Here's how the part is built. I have some questions about the finished solid (model axes, mm). A direction names the side the tool comes from. Round coordinates to 2 decimals unless told otherwise and drop trailing zeros. Loops run counter-clockwise (first coordinate to the right, second up) from the corner with the lowest first, then second, coordinate; pieces in that order, holes last. Notation, with made-up numbers: M -30,15 L -17,15 A31 cw -17,40 Z; hole C 1.5,26.5 d2. An arc over 180 degrees is marked long. Answer as CSV lines item,"result".
```python
from build123d import *
from build123d.topology import SkipClean

# Parameters (mm, degrees)
SKETCH_1_R               = 82.5
SKETCH_1_R_2             = 12.5
EXTRUDE_1_DEPTH          = 5
SKETCH_2_R               = 4
SKETCH_2_R_2             = 3
EXTRUDE_2_DEPTH          = 18
EXTRUDE_START            = 5
SKETCH_3_R               = 35
SKETCH_3_R_2             = 12.5
EXTRUDE_3_DEPTH          = 5
CUT_EXTRUDE_1_DEPTH      = 119.05295422
CUT_EXTRUDE_1_DEPTH_BACK = 10
SKETCH_4_R               = 82.5
EXTRUDE_4_DEPTH          = 5
SKETCH_6_R               = 12.5
CUT_EXTRUDE_2_DEPTH      = 110.399094856
SKETCH_7_R               = 34.75
SKETCH_7_R_2             = 12.5
EXTRUDE_5_DEPTH          = 5


with BuildPart() as part:
    # 草圖1 → 填料-伸長1 (new body)
    with BuildSketch(Plane(origin=(0, 0, 0), x_dir=(1, 0, 0), z_dir=(0, 1, 0))):
        with Locations(Location((0, 0, 0), (0, 0, 270))):
            Circle(SKETCH_1_R)
        with Locations(Location((0, 0, 0), (0, 0, 270))):
            Circle(SKETCH_1_R_2, mode=Mode.SUBTRACT)
    extrude(amount=EXTRUDE_1_DEPTH)

    # 草圖2 → 填料-伸長2 (add)
    # profile 1 of 3: a face of its own
    with BuildSketch(Plane(origin=(0, 5, 0), x_dir=(1, 0, 0), z_dir=(0, 1, 0))):
        with Locations(Location((0, 71.25, 0), (0, 0, 270))):
            Circle(SKETCH_2_R)
        with Locations(Location((0, 71.25, 0), (0, 0, 270))):
            Circle(SKETCH_2_R_2, mode=Mode.SUBTRACT)
    # profile 2 of 3: a face of its own
    with BuildSketch(Plane(origin=(0, 5, 0), x_dir=(1, 0, 0), z_dir=(0, 1, 0))):
        with Locations(Location((61.70431002, -35.625, 0), (0, 0, 270))):
            Circle(SKETCH_2_R)
        with Locations(Location((61.70431002, -35.625, 0), (0, 0, 270))):
            Circle(SKETCH_2_R_2, mode=Mode.SUBTRACT)
    # profile 3 of 3: a face of its own
    with BuildSketch(Plane(origin=(0, 5, 0), x_dir=(1, 0, 0), z_dir=(0, 1, 0))):
        with Locations(Location((-61.70431002, -35.625, 0), (0, 0, 270))):
            Circle(SKETCH_2_R)
        with Locations(Location((-61.70431002, -35.625, 0), (0, 0, 270))):
            Circle(SKETCH_2_R_2, mode=Mode.SUBTRACT)
    extrude(amount=EXTRUDE_2_DEPTH)

    # 草圖3 → 填料-伸長3 (add)
    with SkipClean():  # the faces are left unmerged after this step: merging them gives an invalid solid
        with BuildSketch(Plane.XZ.offset(EXTRUDE_START)):
            with Locations(Location((0, 0, 0), (0, 0, 90))):
                Circle(SKETCH_3_R)
            with Locations(Location((0, 0, 0), (0, 0, 270))):
                Circle(SKETCH_3_R_2, mode=Mode.SUBTRACT)
        extrude(amount=-EXTRUDE_3_DEPTH)

    # 草圖4 → 除料-伸長1 (cut, two sides: drawn at the far end of the back side and taken through both)
    with SkipClean():  # the faces are left unmerged after this step: merging them gives an invalid solid
        with BuildSketch(Plane(origin=(0, 5, 0), x_dir=(1, 0, 0), z_dir=(0, 1, 0)).offset(-CUT_EXTRUDE_1_DEPTH_BACK)):
            Circle(SKETCH_4_R)
            with BuildLine():
                ThreePointArc((-35.334504499, -38.829406277), (0, -52.5), (35.334504499, -38.829406277))
                ThreePointArc((35.334504499, -38.829406277), (40.993396246, -36.283053927), (47.064886308, -37.565229625))
                Line((47.064886308, -37.565229625), (57.20431002, -43.419228634))
                ThreePointArc((57.20431002, -43.419228634), (69.498538654, -40.125), (66.20431002, -27.830771366))
                Line((66.20431002, -27.830771366), (56.064886308, -21.976772357))
                ThreePointArc((56.064886308, -21.976772357), (51.918744551, -17.359795573), (51.294504499, -11.185875388))
                ThreePointArc((51.294504499, -11.185875388), (45.466333699, 26.25), (15.96, 50.015281665))
                ThreePointArc((15.96, 50.015281665), (10.925348305, 53.6428495), (9, 59.542001982))
                Line((9, 59.542001982), (9, 71.25))
                ThreePointArc((9, 71.25), (0, 80.25), (-9, 71.25))
                Line((-9, 71.25), (-9, 59.542001982))
                ThreePointArc((-9, 59.542001982), (-10.925348305, 53.6428495), (-15.96, 50.015281665))
                ThreePointArc((-15.96, 50.015281665), (-45.466333699, 26.25), (-51.294504499, -11.185875388))
                ThreePointArc((-51.294504499, -11.185875388), (-51.918744551, -17.359795573), (-56.064886308, -21.976772357))
                Line((-56.064886308, -21.976772357), (-66.20431002, -27.830771366))
                ThreePointArc((-66.20431002, -27.830771366), (-69.498538654, -40.125), (-57.20431002, -43.419228634))
                Line((-57.20431002, -43.419228634), (-47.064886308, -37.565229625))
                ThreePointArc((-47.064886308, -37.565229625), (-40.993396246, -36.283053927), (-35.334504499, -38.829406277))
            make_face(mode=Mode.SUBTRACT)
        extrude(amount=CUT_EXTRUDE_1_DEPTH + CUT_EXTRUDE_1_DEPTH_BACK, mode=Mode.SUBTRACT)

    # 草圖5 → 填料-伸長4 (add)
    with BuildSketch(Plane.XZ):
        with BuildLine():
            Line((-47.064886308, 37.565229625), (-57.20431002, 43.419228634))
            ThreePointArc((-57.20431002, 43.419228634), (-69.498538654, 40.125), (-66.20431002, 27.830771366))
            Line((-66.20431002, 27.830771366), (-56.064886308, 21.976772357))
            ThreePointArc((-56.064886308, 21.976772357), (-51.918744551, 17.359795573), (-51.294504499, 11.185875388))
            ThreePointArc((-51.294504499, 11.185875388), (-45.466333699, -26.25), (-15.96, -50.015281665))
            ThreePointArc((-15.96, -50.015281665), (-10.925348305, -53.6428495), (-9, -59.542001982))
            Line((-9, -59.542001982), (-9, -71.25))
            ThreePointArc((-9, -71.25), (0, -80.25), (9, -71.25))
            Line((9, -71.25), (9, -59.542001982))
            ThreePointArc((9, -59.542001982), (10.925348305, -53.6428495), (15.96, -50.015281665))
            ThreePointArc((15.96, -50.015281665), (45.466333699, -26.25), (51.294504499, 11.185875388))
            ThreePointArc((51.294504499, 11.185875388), (51.918744551, 17.359795573), (56.064886308, 21.976772357))
            Line((56.064886308, 21.976772357), (66.20431002, 27.830771366))
            ThreePointArc((66.20431002, 27.830771366), (69.498538654, 40.125), (57.20431002, 43.419228634))
            Line((57.20431002, 43.419228634), (47.064886308, 37.565229625))
            ThreePointArc((47.064886308, 37.565229625), (40.993396246, 36.283053927), (35.334504499, 38.829406277))
            ThreePointArc((35.334504499, 38.829406277), (0, 52.5), (-35.334504499, 38.829406277))
            ThreePointArc((-35.334504499, 38.829406277), (-40.993396246, 36.283053927), (-47.064886308, 37.565229625))
        make_face()
    extrude(amount=EXTRUDE_4_DEPTH)

    # 草圖6 → 除料-伸長2 (cut, through all)
    with BuildSketch(Plane(origin=(0, 0, 0), x_dir=(1, 0, 0), z_dir=(0, 1, 0))):
        with Locations(Location((0, 0, 0), (0, 0, 270))):
            Circle(SKETCH_6_R)
    extrude(amount=-CUT_EXTRUDE_2_DEPTH, mode=Mode.SUBTRACT)

    # 草圖7 → 填料-伸長5 (add)
    with SkipClean():  # the faces are left unmerged after this step: merging them gives an invalid solid
        with BuildSketch(Plane.XZ.offset(5)):
            with Locations(Location((0, 0, 0), (0, 0, 270))):
                Circle(SKETCH_7_R)
            with Locations(Location((0, 0, 0), (0, 0, 270))):
                Circle(SKETCH_7_R_2, mode=Mode.SUBTRACT)
        extrude(amount=EXTRUDE_5_DEPTH)
    add(part.part.scale(1), mode=Mode.REPLACE)  # the faces are merged on a copy


solid = part.part
```
1. For P1, Ø8, axis at x = -16.5, z = 15.5, coming from the +Y side; P2, Ø8, axis at x = 0, z = -71.25, coming from the -Y side; P3, Ø11, axis at y = -2, z = -62.5, coming from the +X side; P4, Ø15, axis at x = 0, z = 0, coming from the +Y side, each with a flat end and sliding along its axis, tell me the tip position at first contact or that it passes through.
Evaluation:
P1,"stops at y = 5"
P2,"stops at y = -5"
P3,"stops at x = 9.33"
P4,"passes through"
2. We'd pull the mould along X, two halves only. Please class faces 1 (the cylindrical face through (63.73, 13.87, 33.41)), 2 (the flat face through (9, 0, -65)), 3 (the flat face through (0, -10, -15)), 4 (the cylindrical face through (34.454, -7.465, 4.524)): pulls with the +X half, pulls with the -X half, needs draft (parallel to the pull), parting line crosses it, or undercut.
Evaluation:
face 1,"undercut"
face 2,"pulls with the +X half"
face 3,"needs draft"
face 4,"parting line crosses it"
3. If I drill on line 1 (X direction, y = -6.65, z = 0); line 2 (X direction, y = 1, z = 42.5); line 3 (Z direction, x = 0, y = -3.8), over which ranges is the centre line in solid material (lowest first)? Write a range as [from, to].
Evaluation:
line 1,"x = [-34.75, -12.5], [12.5, 34.75]"
line 2,"x = [-67.51, -55.61], [-30.82, 30.82], [55.61, 67.51]"
line 3,"z = [-80.25, -12.5], [12.5, 52.5]"
4. I want a section at B-B, the plane z = 0. Please give me the cut outline in (x, y).
Evaluation:
outline,"M -52.5,-5 L -34.75,-5 L -34.75,-10 L -12.5,-10 L -12.5,5 L -52.5,5 Z; M 12.5,-10 L 34.75,-10 L 34.75,-5 L 52.5,-5 L 52.5,5 L 12.5,5 Z"
5. I want a section at D-D, the plane x = -24. Please give me the cut outline in (y, z), and give its area (3 significant figures).
Evaluation:
outline,"M -10,-25.13 L -5,-25.13 L -5,-46.69 L 5,-46.69 L 5,46.69 L -5,46.69 L -5,25.13 L -10,25.13 Z"
area,"1,190 mm²"
6. I want a section at A-A, the plane x = 0. Please give me the cut outline in (y, z).
Evaluation:
outline,"M -10,-34.75 L -5,-34.75 L -5,-80.25 L 5,-80.25 L 5,-75.25 L 23,-75.25 L 23,-74.25 L 5,-74.25 L 5,-68.25 L 23,-68.25 L 23,-67.25 L 5,-67.25 L 5,-12.5 L -10,-12.5 Z; M -10,12.5 L 5,12.5 L 5,52.5 L -5,52.5 L -5,34.75 L -10,34.75 Z"
7. Which directions (+Z, -Z, +X, -X, +Y, -Y) give clear straight access to the entire face, cutting with the end or side of a thin tool? Please do faces 5 (the flat face through (-62, 5, 36)), 6 (the flat face through (21, -5, -28)), 7 (the flat face through (-52.06, 0.07, 40.45)).
Evaluation:
face 5,"+Y"
face 6,"-Y"
face 7,"+Z, +Y, -Y"
8. I want a section at C-C, the plane y = 12. Please give me the cut outline in (x, z) (3 decimals), and give its area (3 significant figures).
Evaluation:
outline,"C -61.704,35.625 d8; C 0,-71.25 d8; C 61.704,35.625 d8; hole C -61.704,35.625 d6; hole C 0,-71.25 d6; hole C 61.704,35.625 d6"
area,"66.0 mm²"
